The listing builds one solid part. Answer for the finished solid, in the listing's coordinates (mm). Face numbers are marked on the shaded views. A direction names the side the tool comes from. Coordinates: 2 decimals unless noted, no trailing zeros. Order: outer loops, then holes, each group sorted by start corner. A loop starts at its lowest first (then second) coordinate and runs counter-clockwise, first axis right, second up. Notation, with made-up numbers: (20.5, -2) -> (55.5, -2) arc R14 ccw to (55.5, 10) -> close; hole circle Ø4 at (-13, 56.25). An arc over 180 degrees is marked (long way). Answer in a Markdown table with one row per item.
```python
from build123d import *

# Parameters (mm, degrees)
SALIENTE_EXTRUIR1_DEPTH         = 43.688
CROQUIS2_W                      = 3
CROQUIS2_H                      = 14.32
CORTAR_EXTRUIR1_DEPTH           = 43.688
CROQUIS3_W                      = 30.48
CROQUIS3_H                      = 3.2375
CORTAR_EXTRUIR2_DEPTH           = 43.688
CROQUIS4_R                      = 2.5
SALIENTE_EXTRUIR2_DEPTH         = 31.8125
CROQUIS5_W                      = 45.466
CROQUIS5_H                      = 25.4625
CORTAR_EXTRUIR3_DEPTH           = 43.688
DESPLEGAR_PLIEGUES5_OUTLINE_W   = 91
DESPLEGAR_PLIEGUES5_OUTLINE_H   = 3.175
DESPLEGAR_PLIEGUES5_DEPTH       = 25.4625
DESPLEGAR_START                 = 25.4625
DESPLEGAR_PLIEGUES5_2_OUTLINE_R = 2.5
DESPLEGAR_PLIEGUES5_2_DEPTH     = 3.175
PROCESAR_START                  = -27.639987743
PROCESAR_PLIEGUES5_OUTLINE_W    = 43.688
PROCESAR_PLIEGUES5_OUTLINE_H    = 3.175
PROCESAR_PLIEGUES5_DEPTH        = 24.464987743
PROCESAR_START_2                = 28.6375
PROCESAR_PLIEGUES5_2_OUTLINE_W  = 43.688
PROCESAR_PLIEGUES5_2_OUTLINE_H  = 3.175
PROCESAR_PLIEGUES5_2_DEPTH      = 24.464987743
PROCESAR_START_3                = -3.175
PROCESAR_PLIEGUES5_3_OUTLINE_R  = 2.5
PROCESAR_PLIEGUES5_3_DEPTH      = 3.9116
PROCESAR_START_4                = 24.7259
PROCESAR_PLIEGUES5_4_OUTLINE_R  = 2.5
PROCESAR_PLIEGUES5_4_DEPTH      = 3.9116
PROCESAR_PLIEGUES5_5_OUTLINE_W  = 3.175
PROCESAR_PLIEGUES5_5_OUTLINE_H  = 14.224
PROCESAR_PLIEGUES5_5_DEPTH      = 90


with BuildPart() as part:
    # Croquis1 → Saliente-Extruir1 (new body)
    with BuildSketch(Plane(origin=(0, 0, 0), x_dir=(0, 0, -1), z_dir=(1, 0, 0))):
        Polygon((-28.6375, 0), (-28.6375, 28.6375), (3.175, 28.6375), (3.175, 0), (0, 0), (0, 25.4625), (-25.4625, 25.4625), (-25.4625, 0), align=None)
    extrude(amount=SALIENTE_EXTRUIR1_DEPTH)

    # Croquis2 → Cortar-Extruir1 (cut)
    with BuildSketch(Plane.XY.offset(28.6375)):
        with Locations((1.5, 7.16)):
            Rectangle(CROQUIS2_W, CROQUIS2_H)
    extrude(amount=-CORTAR_EXTRUIR1_DEPTH, mode=Mode.SUBTRACT)

    # Croquis3 → Cortar-Extruir2 (cut)
    with BuildSketch(Plane(origin=(0, 28.6375, 0), x_dir=(1, 0, 0), z_dir=(0, 1, 0))):
        with Locations((21.844, -12.73125)):
            Rectangle(CROQUIS3_W, CROQUIS3_H)
    extrude(amount=-CORTAR_EXTRUIR2_DEPTH, mode=Mode.SUBTRACT)

    # Croquis4 → Saliente-Extruir2 (add)
    with BuildSketch(Plane.XY.offset(28.6375)):
        with BuildLine():
            Line((43.688, 14.224), (82.042, 14.224))
            ThreePointArc((82.042, 14.224), (89.154, 7.112), (82.042, 0))
            Line((82.042, 0), (43.688, 0))
            Line((43.688, 0), (43.688, 14.224))
        make_face()
        with Locations((82.042, 7.112)):
            Circle(CROQUIS4_R, mode=Mode.SUBTRACT)
    extrude(amount=-SALIENTE_EXTRUIR2_DEPTH)

    # Croquis5 → Cortar-Extruir3 (cut)
    with BuildSketch(Plane(origin=(0, 14.224, 0), x_dir=(1, 0, 0), z_dir=(0, 1, 0))):
        with Locations((66.421, -12.73125)):
            Rectangle(CROQUIS5_W, CROQUIS5_H)
    extrude(amount=-CORTAR_EXTRUIR3_DEPTH, mode=Mode.SUBTRACT)

    # Desplegar pliegues5: read off the stored shape, not the designer's step
    # Desplegar pliegues5 outline → Desplegar pliegues5 (cut)
    with BuildSketch(Plane(origin=(0, 0, 0), x_dir=(1, 0, 0), z_dir=(0, 1, 0))):
        with Locations((45.5, -27.05)):
            Rectangle(DESPLEGAR_PLIEGUES5_OUTLINE_W, DESPLEGAR_PLIEGUES5_OUTLINE_H)
        with Locations((45.5, 1.5875)):
            Rectangle(DESPLEGAR_PLIEGUES5_OUTLINE_W, DESPLEGAR_PLIEGUES5_OUTLINE_H)
    extrude(amount=DESPLEGAR_PLIEGUES5_DEPTH, mode=Mode.SUBTRACT)

    # Desplegar pliegues5 2 outline → Desplegar pliegues5 2 (add)
    # profile 1 of 2: a face of its own
    with BuildSketch(Plane(origin=(0, 0, 0), x_dir=(1, 0, 0), z_dir=(0, 1, 0)).offset(DESPLEGAR_START)):
        with BuildLine():
            Line((0, -28.6375), (0, -38.782487743))
            Line((0, -38.782487743), (3, -38.782487743))
            Line((3, -38.782487743), (3, -53.102487743))
            Line((3, -53.102487743), (82.042, -53.102487743))
            ThreePointArc((82.042, -53.102487743), (89.154, -45.990487743), (82.042, -38.878487743))
            Line((82.042, -38.878487743), (43.688, -38.878487743))
            Line((43.688, -38.878487743), (43.688, -28.6375))
            Line((43.688, -28.6375), (0, -28.6375))
        make_face()
        with Locations((82.042, -45.990487743)):
            Circle(DESPLEGAR_PLIEGUES5_2_OUTLINE_R, mode=Mode.SUBTRACT)
    # profile 2 of 2: a face of its own
    with BuildSketch(Plane(origin=(0, 0, 0), x_dir=(1, 0, 0), z_dir=(0, 1, 0)).offset(DESPLEGAR_START)):
        with BuildLine():
            Line((3, 27.639987743), (3, 13.319987743))
            Line((3, 13.319987743), (0, 13.319987743))
            Line((0, 13.319987743), (0, 3.175))
            Line((0, 3.175), (43.688, 3.175))
            Line((43.688, 3.175), (43.688, 13.415987743))
            Line((43.688, 13.415987743), (82.042, 13.415987743))
            ThreePointArc((82.042, 13.415987743), (89.154, 20.527987743), (82.042, 27.639987743))
            Line((82.042, 27.639987743), (3, 27.639987743))
        make_face()
        with Locations((82.042, 20.527987743)):
            Circle(DESPLEGAR_PLIEGUES5_2_OUTLINE_R, mode=Mode.SUBTRACT)
    extrude(amount=DESPLEGAR_PLIEGUES5_2_DEPTH)

    # Procesar pliegues5: read off the stored shape, not the designer's step
    # Procesar pliegues5 outline → Procesar pliegues5 (cut)
    with BuildSketch(Plane.XY.offset(PROCESAR_START)):
        with Locations((21.844, 27.05)):
            Rectangle(PROCESAR_PLIEGUES5_OUTLINE_W, PROCESAR_PLIEGUES5_OUTLINE_H)
    extrude(amount=PROCESAR_PLIEGUES5_DEPTH, mode=Mode.SUBTRACT)

    # Procesar pliegues5 2 outline → Procesar pliegues5 2 (cut)
    with BuildSketch(Plane.XY.offset(PROCESAR_START_2)):
        with Locations((21.844, 27.05)):
            Rectangle(PROCESAR_PLIEGUES5_2_OUTLINE_W, PROCESAR_PLIEGUES5_2_OUTLINE_H)
    extrude(amount=PROCESAR_PLIEGUES5_2_DEPTH, mode=Mode.SUBTRACT)

    # Procesar pliegues5 3 outline → Procesar pliegues5 3 (add)
    with BuildSketch(Plane.XY.offset(PROCESAR_START_3)):
        with BuildLine():
            Line((3, 14.32), (3, 0))
            Line((3, 0), (82.042, 0))
            ThreePointArc((82.042, 0), (89.154, 7.112), (82.042, 14.224))
            Line((82.042, 14.224), (43.688, 14.224))
            Line((43.688, 14.224), (43.688, 25.4625))
            Line((43.688, 25.4625), (0, 25.4625))
            Line((0, 25.4625), (0, 14.32))
            Line((0, 14.32), (3, 14.32))
        make_face()
        with Locations((82.042, 7.112)):
            Circle(PROCESAR_PLIEGUES5_3_OUTLINE_R, mode=Mode.SUBTRACT)
    extrude(amount=PROCESAR_PLIEGUES5_3_DEPTH)

    # Procesar pliegues5 4 outline → Procesar pliegues5 4 (add)
    with BuildSketch(Plane.XY.offset(PROCESAR_START_4)):
        with BuildLine():
            Line((3, 14.32), (3, 0))
            Line((3, 0), (82.042, 0))
            ThreePointArc((82.042, 0), (89.154, 7.112), (82.042, 14.224))
            Line((82.042, 14.224), (43.688, 14.224))
            Line((43.688, 14.224), (43.688, 25.4625))
            Line((43.688, 25.4625), (0, 25.4625))
            Line((0, 25.4625), (0, 14.32))
            Line((0, 14.32), (3, 14.32))
        make_face()
        with Locations((82.042, 7.112)):
            Circle(PROCESAR_PLIEGUES5_4_OUTLINE_R, mode=Mode.SUBTRACT)
    extrude(amount=PROCESAR_PLIEGUES5_4_DEPTH)

    # Procesar pliegues5 5 outline → Procesar pliegues5 5 (cut)
    with BuildSketch(Plane.YZ):
        with BuildLine():
            Line((0, 0.7366), (0, 0))
            Line((0, 0), (24.7259, 0))
            ThreePointArc((24.7259, 0), (25.246754855, 0.215745145), (25.4625, 0.7366))
            Line((25.4625, 0.7366), (0, 0.7366))
        make_face()
        with BuildLine():
            ThreePointArc((24.7259, 28.6375), (27.491818885, 27.491818885), (28.6375, 24.7259))
            Line((28.6375, 24.7259), (28.6375, 28.6375))
            Line((28.6375, 28.6375), (24.7259, 28.6375))
        make_face()
        with BuildLine():
            ThreePointArc((28.6375, 0.7366), (27.491818885, -2.029318885), (24.7259, -3.175))
            Line((24.7259, -3.175), (28.6375, -3.175))
            Line((28.6375, -3.175), (28.6375, 0.7366))
        make_face()
        with BuildLine():
            ThreePointArc((25.4625, 24.7259), (25.246754855, 25.246754855), (24.7259, 25.4625))
            Line((24.7259, 25.4625), (0, 25.4625))
            Line((0, 25.4625), (0, 24.7259))
            Line((0, 24.7259), (25.4625, 24.7259))
        make_face()
        with Locations((27.05, 45.990487743)):
            Rectangle(PROCESAR_PLIEGUES5_5_OUTLINE_W, PROCESAR_PLIEGUES5_5_OUTLINE_H)
        with Locations((27.05, -20.527987743)):
            Rectangle(PROCESAR_PLIEGUES5_5_OUTLINE_W, PROCESAR_PLIEGUES5_5_OUTLINE_H)
    extrude(amount=PROCESAR_PLIEGUES5_5_DEPTH, mode=Mode.SUBTRACT)


solid = part.part
```
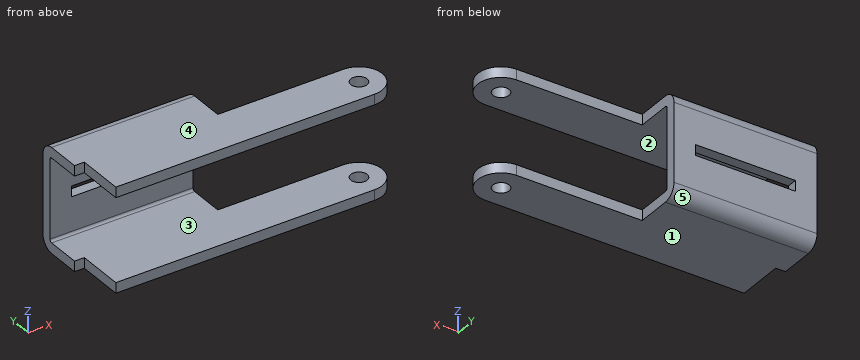
(1) Find the intervals of material crossed by line 1 along Z through (x, y) = (22, 17.25) (1 decimal); line 2 along Y through (x, z) = (8, 16.5); line 3 along X through (y, z) = (23.5, 26), in increasing order. Write a range as from..to.
Check values:
| item | result |
|---|---|
| line 1 | -3.2..0, 25.5..28.6 |
| line 2 | 25.46..28.64 |
| line 3 | 0..43.69 |
(2) A cutting plane is placed at A-A, the plane y = 17.75. Determine the outline of the cut face in (x, z) (1 decimal), then the cut area to 3 significant figures.
Check values:
| item | result |
|---|---|
| outline | (0, -3.2) -> (43.7, -3.2) -> (43.7, 0) -> (0, 0) -> close; (0, 25.5) -> (43.7, 25.5) -> (43.7, 28.6) -> (0, 28.6) -> close |
| area | 277 mm² |
(3) A cutting plane is placed at D-D, the plane y = 5.5. Determine the outline of the cut face in (x, z) (1 decimal).
Check values:
| item | result |
|---|---|
| outline | (3, -3.2) -> (80.1, -3.2) -> (80.1, 0) -> (3, 0) -> close; (3, 25.5) -> (80.1, 25.5) -> (80.1, 28.6) -> (3, 28.6) -> close; (84, -3.2) -> (89, -3.2) -> (89, 0) -> (84, 0) -> close; (84, 25.5) -> (89, 25.5) -> (89, 28.6) -> (84, 28.6) -> close |
(4) Flat-ended cylindrical pins translate along their axes: pin 1 (7 mm diameter, centred on x = 20, z = 7, fed in from -Y); pin 2 (0.9 mm diameter, centred on x = 2, z = 27, fed in from -Y); pin 3 (1.6 mm diameter, centred on x = 63.5, z = 27.5, fed in from +Y). Find the tip coordinate at first contact, or state that the pin passes through.
Check values:
| item | result |
|---|---|
| pin 1 | y = 25.46 |
| pin 2 | y = 14.32 |
| pin 3 | y = 14.22 |
(5) A cutting plane is placed at C-C, the plane z = 13. Determine the outline of the cut face in (x, y), then the cut area to 3 significant figures.
Check values:
| item | result |
|---|---|
| outline | (0, 25.46) -> (6.6, 25.46) -> (6.6, 28.64) -> (0, 28.64) -> close; (37.08, 25.46) -> (43.69, 25.46) -> (43.69, 28.64) -> (37.08, 28.64) -> close |
| area | 41.9 mm² |
(6) For a pull along Z with two mould halves and no side action, classify the marked faces 3, 4 and 5 as released by +Z, released by -Z, zero draft, split by the parting line, or undercut.
Check values:
| item | result |
|---|---|
| face 3 | undercut |
| face 4 | released by +Z |
| face 5 | released by -Z |
(7) Which of the six approach directions +Z, -Z, +X, -X, +Y, -Y give full straight-line access (tool end or side, diameter ignored) to the marked faces 1 and 2?
Check values:
| item | result |
|---|---|
| face 1 | -Z, +X, -X, +Y, -Y |
| face 2 | +X, -X, -Y |
